from build123d import *

# Parameters (mm, degrees)
F0_R     = 1.5
F1_DEPTH = 4.7625


with BuildPart() as f1:
    # F0 (on Front) → F1 (new body)
    with BuildSketch(Plane.XZ):
        with BuildLine():
            Line((10.109961, -9.738645), (10.109961, -11.715053))
            ThreePointArc((10.109961, -11.715053), (12.991369, -8.203415), (14.699125, -3.994177))
            Line((14.699125, -3.994177), (0, 2.9986))
            Line((0, 2.9986), (-14.699125, -3.994177))
            ThreePointArc((-14.699125, -3.994177), (-13.361828, -7.543024), (-11.183127, -10.647207))
            Line((-11.183127, -10.647207), (-9.269246, -10.580372))
            ThreePointArc((-9.269246, -10.580372), (-11.57614, -7.823081), (-13.086808, -4.560827))
            Line((-13.086808, -4.560827), (0, -3.0014))
            Line((0, -3.0014), (13.086808, -4.560827))
            ThreePointArc((13.086808, -4.560827), (11.883812, -7.313834), (10.109961, -9.738645))
        make_face()
        Circle(F0_R, mode=Mode.SUBTRACT)
    extrude(amount=F1_DEPTH)


solid = f1.part
Check sheet for the modelled part. Datum: model origin and axes. Units: mm. A direction names the side the tool comes from. Coordinates: 2 decimals unless noted, no trailing zeros. Write each loop counter-clockwise with the first axis right and the second up, starting at its lowest first coordinate (ties: lowest second). Pieces come first, ordered by that corner, then holes.
Item 1: Cross-section at A-A on y = -1.4. Record the boundary of the cut face in (x, z).
Numbers:
outline: (-14.7, -3.99) arc R15.11 ccw to (-11.18, -10.65) - (-9.27, -10.58) arc R13.71 cw to (-13.09, -4.56) - (0, -3) - (13.09, -4.56) arc R13.71 cw to (10.11, -9.74) - (10.11, -11.72) arc R15.11 ccw to (14.7, -3.99) - (0, 3) - close; hole circle Ø3 at (0, 0)
Item 2: Cross-section at C-C on x = -12.75. Record the boundary of the cut face in (y, z), then the cut area to 3 significant figures.
Numbers:
outline: (-4.76, -8.6) - (0, -8.6) - (0, -5.52) - (-4.76, -5.52) - close; (-4.76, -4.52) - (0, -4.52) - (0, -3.07) - (-4.76, -3.07) - close
area: 21.6 mm2
Item 3: Cross-section at B-B on z = -5. Record the boundary of the cut face in (x, y).
Numbers:
outline: (-14.42, -4.76) - (-12.94, -4.76) - (-12.94, 0) - (-14.42, 0) - close; (12.94, -4.76) - (14.42, -4.76) - (14.42, 0) - (12.94, 0) - close
Item 4: Access from +Z, -Z, +X, -X, +Y, -Y to the whole of each face (thin tool, end or side, straight path). Record for faces 1 (the face through (-7.25, -2.35, -0.45)), 2 (the face through (10.11, -2, -11)), 3 (the face through (6.45, -2.35, -3.77)).
Numbers:
face 1: +Z, -X, +Y, -Y
face 2: -Z, +Y, -Y
face 3: +Y, -Y
Item 5: Cross-section at D-D on x = -5.5. Record the boundary of the cut face in (y, z).
Numbers:
outline: (-4.76, -3.66) - (0, -3.66) - (0, 0.38) - (-4.76, 0.38) - close
Item 6: Scan lines: probe 1 along Z at (x, y) = (0, -1.8); probe 2 along X at (y, z) = (-0.25, -8.5); probe 3 along Z at (x, y) = (11.5, -4.35). Record each from-to range of solid material in increasing order.
Numbers:
probe 1: z = -3 to -1.5, 1.5 to 3
probe 2: x = -12.81 to -11.12, 11.12 to 12.81
probe 3: z = -10.29 to -7.94, -4.37 to -2.47
Item 7: Depth check by flat-ended pin: pin 1 Ø4 at (x, z) = (0, 0) entering from -Y; pin 2 Ø0.6 at (y, z) = (-1.5, -11) entering from -X. Enter the tip coordinate at first touch or a pass-through.
Numbers:
pin 1: stops at y = -4.76
pin 2: stops at x = 10.11
Item 8: Mould release check, pull along X, two halves, no side actions. Record for faces 4 (the face through (-13.387, -2.348, -7.496)), 5 (the face through (7.452, -2.348, -0.547)), 6 (the face through (0, 0, -2)), 7 (the face through (11.905, -2.348, -7.277)): released by +X, released by -X, zero draft, split by the parting line, or undercut.
Numbers:
face 4: released by -X
face 5: released by +X
face 6: zero draft
face 7: undercut
